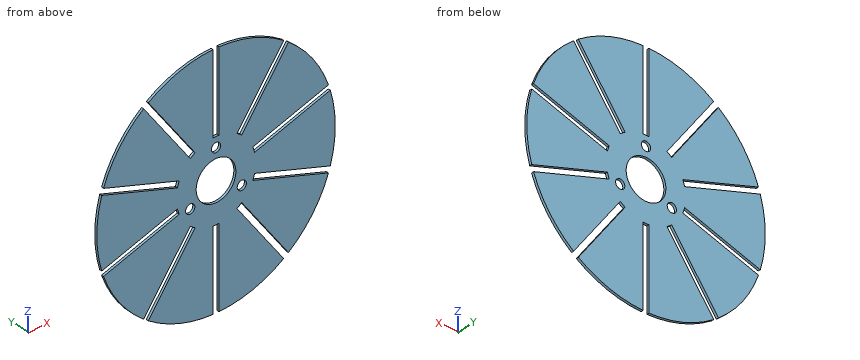
```python
from build123d import *

# Parameters (mm, degrees)
F0_R            = 38.1
F0_R_2          = 6.35
F1_DEPTH        = 0.762
F3_DEPTH        = 0.763
F3_COPIES_COUNT = 10
F5_D            = 2.9464


# Not quite as in the source:
# - a pattern or mirror of a feature is missing from the dataset's text; its kind, count and spacing are read off the source's solid


with BuildPart() as f1:
    # F0 (on Front) → F1 (new body)
    with BuildSketch(Plane.XZ):
        Circle(F0_R)
        Circle(F0_R_2, mode=Mode.SUBTRACT)
    extrude(amount=F1_DEPTH)

    # F2 (on face) → F3 (cut, through all)
    with BuildSketch(Plane.XZ.offset(0.762)):
        with BuildLine():
            Line((-0.9345413193, 38.0885367601), (-0.9345413193, 12.6655687801))
            ThreePointArc((-0.9345413193, 12.6655687801), (0, 12.7), (0.9345413193, 12.6655687801))
            Line((0.9345413193, 12.6655687801), (0.9345413193, 38.0885367601))
            ThreePointArc((0.9345413193, 38.0885367601), (0, 38.1), (-0.9345413193, 38.0885367601))
        make_face()
    f3 = extrude(amount=-F3_DEPTH, mode=Mode.SUBTRACT)

    # F3_copies: F3 ×10 about axis
    f3_copies_axis = Axis((0, 0, 0), (0, 1, 0))
    for i in range(1, F3_COPIES_COUNT):
        add(f3.rotate(f3_copies_axis, i * 360 / F3_COPIES_COUNT), mode=Mode.SUBTRACT)

    # F5 (through all)
    with Locations(Plane.XZ.offset(0.762)):
        with Locations((0, 9.525), (-8.248891971, -4.7625), (8.248891971, -4.7625)):
            Hole(F5_D / 2)


solid = f1.part
```
CAD build for the part. Positions are in the model's coordinates, mm. Give positions to 0.01 mm unless a question says otherwise; leave off trailing zeros. Loops run counter-clockwise (first coordinate to the right, second up) from the corner with the lowest first, then second, coordinate; pieces in that order, holes last. Notation, with made-up numbers: (31, -7) -> (39, -7) arc R17 cw to (39, 11) -> close; hole circle Ø3 at (49, 21). An arc over 180 degrees is marked (long way). Use a Markdown table: item, result.
1. Slice it at D-D (x = 24.5). List the corners of the cut face in (y, z).
Check result:
| item | result |
|---|---|
| outline | (-0.76, -29.18) -> (0, -29.18) -> (0, -8.94) -> (-0.76, -8.94) -> close; (-0.76, -6.98) -> (0, -6.98) -> (0, 6.98) -> (-0.76, 6.98) -> close; (-0.76, 8.94) -> (0, 8.94) -> (0, 29.18) -> (-0.76, 29.18) -> close |
2. Wall check: L1, parallel to Z at x = 0, y = -0.5; L2, parallel to Z at x = -19, y = -0.55; L3, parallel to Z at x = -33, y = -0.5. Give the ranges that are in metal, low to high. Write a range as [from, to].
Check result:
| item | result |
|---|---|
| L1 | z = [-12.7, -6.35], [6.35, 8.05], [11, 12.7] |
| L2 | z = [-33.02, -27.74], [-24.56, -7.16], [-5.19, 5.19], [7.16, 24.56], [27.74, 33.02] |
| L3 | z = [-19.04, -11.7], [-9.74, 9.74], [11.7, 19.04] |
3. Flat gauge pins, fed straight in: pin 1 (4.5 mm diameter, centred on x = -8.25, z = -4.76, fed in from +Y); pin 2 (10 mm diameter, centred on x = 0.5, z = 1, fed in from -Y). Where does each tip first touch, or does it go through?
Check result:
| item | result |
|---|---|
| pin 1 | stops at y = 0 |
| pin 2 | passes through |
4. Slice it at C-C (z = 22.5). List the corners of the cut face in (x, y).
Check result:
| item | result |
|---|---|
| outline | (-30.75, -0.76) -> (-17.5, -0.76) -> (-17.5, 0) -> (-30.75, 0) -> close; (-15.19, -0.76) -> (-0.93, -0.76) -> (-0.93, 0) -> (-15.19, 0) -> close; (0.93, -0.76) -> (15.19, -0.76) -> (15.19, 0) -> (0.93, 0) -> close; (17.5, -0.76) -> (30.75, -0.76) -> (30.75, 0) -> (17.5, 0) -> close |
5. Slice it at A-A (z = 0). List the corners of the cut face in (x, y).
Check result:
| item | result |
|---|---|
| outline | (-38.1, -0.76) -> (-6.35, -0.76) -> (-6.35, 0) -> (-38.1, 0) -> close; (6.35, -0.76) -> (38.1, -0.76) -> (38.1, 0) -> (6.35, 0) -> close |
6. Slice it at B-B (x = 0). List the corners of the cut face in (y, z).
Check result:
| item | result |
|---|---|
| outline | (-0.76, -12.7) -> (0, -12.7) -> (0, -6.35) -> (-0.76, -6.35) -> close; (-0.76, 6.35) -> (0, 6.35) -> (0, 8.05) -> (-0.76, 8.05) -> close; (-0.76, 11) -> (0, 11) -> (0, 12.7) -> (-0.76, 12.7) -> close |
